```python
from build123d import *

# Parameters (mm, degrees)
SKETCH1_R                      = 127
BASE_OF_BASE_DEPTH             = 8.89
BALL_BEARING_CUT_REACH         = 221.212
SKETCH8_R                      = 26.035
SUPPORT_REACH                  = 208.429
SUPPORTS_COUNT                 = 4
CUT_FOR_PRINTABIITY_REACH      = 221.212
HOLDER_START                   = 76.2
SKETCH14_R                     = 26.035
SKETCH14_R_2                   = 13.335
HOLDER_FOR_SHOULDER_DEPTH      = 76.2
CENTER_CYLINDER_REACH          = 208.429
SKETCH14_3_R                   = 31.75
SKETCH14_3_R_2                 = 26.035
FUNNEL_INTO_SNAP_IN_PLACE_SIZE = 2.54
ACCESSIBILITY_CUT_DEPTH        = 290.1712073


with BuildPart() as part:
    # Sketch1 → Base of base (new body)
    with BuildSketch(Plane(origin=(0, 0, 0), x_dir=(1, 0, 0), z_dir=(0, 1, 0))):
        with Locations(Location((0, 0, 0), (0, 0, 270))):
            Circle(SKETCH1_R)
    extrude(amount=BASE_OF_BASE_DEPTH)



with BuildPart() as body_2:
    # Sketch7 → Top Part of Base (revolve)
    with BuildSketch(Plane(origin=(0, 0, 0), x_dir=(0, 0, -1), z_dir=(1, 0, 0)), mode=Mode.PRIVATE) as top_part_of_base_sk:
        Polygon((0, 125.681135768), (0, 112.981135768), (-114.3, 46.99), (-114.3, 59.69), align=None)
    revolve(top_part_of_base_sk.sketch.rotate(Axis((0, 8.89, 0), (0, 1, 0)), 180), axis=Axis((0, 8.89, 0), (0, 1, 0)))

    # Ball Bearing Cut: up to this cone (the profile starts outside it)
    ball_bearing_cut_end = Plane(origin=(0, 125.681136, 0), z_dir=(0, -1, 0)).offset(12.700001232) * Cone(1.732e-06, 362.01940299, 209.011998768, align=(Align.CENTER, Align.CENTER, Align.MIN), mode=Mode.PRIVATE)
    # Sketch8 → Ball Bearing Cut (cut, up to the surface)
    with BuildSketch(Plane(origin=(0, 125.681135768, 0), x_dir=(1, 0, 0), z_dir=(0, 1, 0)), mode=Mode.PRIVATE) as ball_bearing_cut_sk1:
        with Locations(Location((0, 0, 0), (0, 0, 90))):
            Circle(SKETCH8_R)
    ball_bearing_cut_tool1 = extrude(ball_bearing_cut_sk1.sketch, amount=-BALL_BEARING_CUT_REACH, mode=Mode.PRIVATE) - ball_bearing_cut_end
    add(ball_bearing_cut_tool1.solids().sort_by_distance((0, 125.681136, 0))[0], mode=Mode.SUBTRACT)


with BuildPart() as part_1:
    add(part.part)

    add(body_2.part)  # Support merges body 2
    # Support: up to this cone (the profile starts inside it)
    support_end = Plane(origin=(0, 8.89, 0), z_dir=(0, -1, 0)).offset(-104.091134768) * Cone(1.732e-06, 854.440186248, 493.311270537, align=(Align.CENTER, Align.CENTER, Align.MIN), mode=Mode.PRIVATE)
    # Sketch10 → Support (add, up to the surface)
    with BuildSketch(Plane(origin=(0, 8.89, 0), x_dir=(1, 0, 0), z_dir=(0, 1, 0)), mode=Mode.PRIVATE) as support_sk1:
        with BuildLine():
            ThreePointArc((-8.301584497, 94.887544993), (-4.154746647, 95.159343106), (0, 95.25))
            Line((0, 95.25), (0, 114.3))
            ThreePointArc((0, 114.3), (-4.985695976, 114.191211727), (-9.961901396, 113.865053992))
            Line((-9.961901396, 113.865053992), (-8.301584497, 94.887544993))
        make_face()
    support_tool1 = extrude(support_sk1.sketch, amount=SUPPORT_REACH, mode=Mode.PRIVATE) & support_end
    # Sketch10 → Support (add, up to the surface)
    with BuildSketch(Plane(origin=(0, 8.89, 0), x_dir=(1, 0, 0), z_dir=(0, 1, 0)), mode=Mode.PRIVATE) as support_sk2:
        with BuildLine():
            Line((0, 114.3), (0, 95.25))
            ThreePointArc((0, 95.25), (4.154746647, 95.159343106), (8.301584497, 94.887544993))
            Line((8.301584497, 94.887544993), (9.961901396, 113.865053992))
            ThreePointArc((9.961901396, 113.865053992), (4.985695976, 114.191211727), (0, 114.3))
        make_face()
    support_tool2 = extrude(support_sk2.sketch, amount=SUPPORT_REACH, mode=Mode.PRIVATE) & support_end
    support = support_tool1.solids().sort_by_distance((-4.581357, 8.89, -104.930336))[0] + support_tool2.solids().sort_by_distance((4.581357, 8.89, -104.930336))[0]
    add(support)

    # Supports: Support ×4 about axis
    supports_axis = Axis((0, 8.89, 0), (0, 1, 0))
    for i in range(1, SUPPORTS_COUNT):
        add(support.rotate(supports_axis, i * 360 / SUPPORTS_COUNT))

    # Cut for Printabiity: up to this cone (the profile starts outside it)
    cut_for_printabiity_end = Plane(origin=(0, 125.681136, 0), z_dir=(0, -1, 0)).offset(12.700001232) * Cone(1.732e-06, 362.01940299, 209.011998768, align=(Align.CENTER, Align.CENTER, Align.MIN), mode=Mode.PRIVATE)
    # Sketch12 → Cut for Printabiity (cut, up to the surface)
    with BuildSketch(Plane(origin=(0, 125.681135768, 0), x_dir=(1, 0, 0), z_dir=(0, 1, 0)), mode=Mode.PRIVATE) as cut_for_printabiity_sk1:
        with BuildLine():
            ThreePointArc((-113.865053992, -9.961901396), (-40.394430205, -40.394430205), (-9.961901396, -113.865053992))
            ThreePointArc((-9.961901396, -113.865053992), (-80.82230509, -80.82230509), (-113.865053992, -9.961901396))
        make_face()
    cut_for_printabiity_tool1 = extrude(cut_for_printabiity_sk1.sketch, amount=-CUT_FOR_PRINTABIITY_REACH, mode=Mode.PRIVATE) - cut_for_printabiity_end
    add(cut_for_printabiity_tool1.solids().sort_by_distance((-60.814886, 125.681136, 60.814886))[0], mode=Mode.SUBTRACT)
    # Sketch12 → Cut for Printabiity (cut, up to the surface)
    with BuildSketch(Plane(origin=(0, 125.681135768, 0), x_dir=(1, 0, 0), z_dir=(0, 1, 0)), mode=Mode.PRIVATE) as cut_for_printabiity_sk2:
        with BuildLine():
            ThreePointArc((-9.961901396, 113.865053992), (-40.394430205, 40.394430205), (-113.865053992, 9.961901396))
            ThreePointArc((-113.865053992, 9.961901396), (-80.82230509, 80.82230509), (-9.961901396, 113.865053992))
        make_face()
    cut_for_printabiity_tool2 = extrude(cut_for_printabiity_sk2.sketch, amount=-CUT_FOR_PRINTABIITY_REACH, mode=Mode.PRIVATE) - cut_for_printabiity_end
    add(cut_for_printabiity_tool2.solids().sort_by_distance((-60.814886, 125.681136, -60.814886))[0], mode=Mode.SUBTRACT)
    # Sketch12 → Cut for Printabiity (cut, up to the surface)
    with BuildSketch(Plane(origin=(0, 125.681135768, 0), x_dir=(1, 0, 0), z_dir=(0, 1, 0)), mode=Mode.PRIVATE) as cut_for_printabiity_sk3:
        with BuildLine():
            ThreePointArc((9.961901396, 113.865053992), (40.394430205, 40.394430205), (113.865053992, 9.961901396))
            ThreePointArc((113.865053992, 9.961901396), (80.82230509, 80.82230509), (9.961901396, 113.865053992))
        make_face()
    cut_for_printabiity_tool3 = extrude(cut_for_printabiity_sk3.sketch, amount=-CUT_FOR_PRINTABIITY_REACH, mode=Mode.PRIVATE) - cut_for_printabiity_end
    add(cut_for_printabiity_tool3.solids().sort_by_distance((60.814886, 125.681136, -60.814886))[0], mode=Mode.SUBTRACT)
    # Sketch12 → Cut for Printabiity (cut, up to the surface)
    with BuildSketch(Plane(origin=(0, 125.681135768, 0), x_dir=(1, 0, 0), z_dir=(0, 1, 0)), mode=Mode.PRIVATE) as cut_for_printabiity_sk4:
        with BuildLine():
            ThreePointArc((9.961901396, -113.865053992), (40.394430205, -40.394430205), (113.865053992, -9.961901396))
            ThreePointArc((113.865053992, -9.961901396), (80.82230509, -80.82230509), (9.961901396, -113.865053992))
        make_face()
    cut_for_printabiity_tool4 = extrude(cut_for_printabiity_sk4.sketch, amount=-CUT_FOR_PRINTABIITY_REACH, mode=Mode.PRIVATE) - cut_for_printabiity_end
    add(cut_for_printabiity_tool4.solids().sort_by_distance((60.814886, 125.681136, 60.814886))[0], mode=Mode.SUBTRACT)

    # Sketch14 → Holder for Shoulder (add)
    with BuildSketch(Plane(origin=(0, 8.89, 0), x_dir=(1, 0, 0), z_dir=(0, 1, 0)).offset(HOLDER_START)):
        with Locations(Location((0, 0, 0), (0, 0, 90))):
            Circle(SKETCH14_R)
        with Locations(Location((0, 0, 0), (0, 0, 90))):
            Circle(SKETCH14_R_2, mode=Mode.SUBTRACT)
    extrude(amount=-HOLDER_FOR_SHOULDER_DEPTH)

    # Center Cylinder: up to this cone (the profile starts inside it)
    center_cylinder_end = Plane(origin=(0, 8.89, 0), z_dir=(0, -1, 0)).offset(-104.091134768) * Cone(1.732e-06, 854.440186248, 493.311270537, align=(Align.CENTER, Align.CENTER, Align.MIN), mode=Mode.PRIVATE)
    # Sketch14<3> → Center Cylinder (add, up to the surface)
    with BuildSketch(Plane(origin=(0, 8.89, 0), x_dir=(1, 0, 0), z_dir=(0, 1, 0)), mode=Mode.PRIVATE) as center_cylinder_sk1:
        with Locations(Location((0, 0, 0), (0, 0, 90))):
            Circle(SKETCH14_3_R)
        with Locations(Location((0, 0, 0), (0, 0, 270))):
            Circle(SKETCH14_3_R_2, mode=Mode.SUBTRACT)
    center_cylinder_tool1 = extrude(center_cylinder_sk1.sketch, amount=CENTER_CYLINDER_REACH, mode=Mode.PRIVATE) & center_cylinder_end
    add(center_cylinder_tool1.solids().sort_by_distance((0, 8.89, 30.851974))[0])

    # Funnel into Snap in Place
    funnel_into_snap_in_place_edges = [part_1.edges().sort_by_distance(p)[0] for p in [
        (0, 85.09, 13.335),
    ]]
    chamfer(funnel_into_snap_in_place_edges, length=FUNNEL_INTO_SNAP_IN_PLACE_SIZE)

    # Sketch19 → Accessibility Cut (cut, through all)
    with BuildSketch(Plane(origin=(-61.913477694, 0, 61.913477694), x_dir=(-0.7071067811865487, 0, -0.7071067811865465), z_dir=(0.7071067811865465, 0, -0.7071067811865487))):
        Polygon((0, 8.89), (15.875, 8.89), (15.875, 43.815), (0, 59.69), (-15.875, 43.815), (-15.875, 8.89), align=None)
    extrude(amount=ACCESSIBILITY_CUT_DEPTH, mode=Mode.SUBTRACT)

    # Sketch20 → Cut-Revolve1 (revolve, cut)
    with BuildSketch(Plane(origin=(0, 0, 0), x_dir=(0, 0, -1), z_dir=(1, 0, 0))):
        Polygon((13.335, 74.295), (13.335, 79.375), (15.875, 79.375), align=None)
    revolve(axis=Axis((0, 8.89, 0), (0, 1, 0)), mode=Mode.SUBTRACT)


solid = part_1.part
```
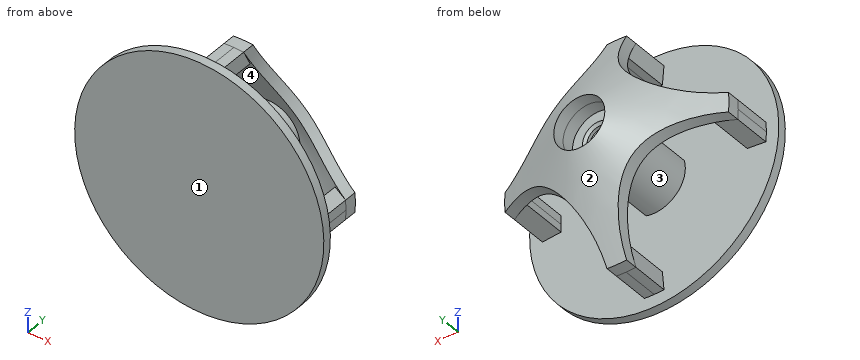
Geometry: final body of the model. Coordinates: model frame, mm. Face numbers are marked on the shaded views. Round coordinates to 2 decimals unless told otherwise and drop trailing zeros. Write each loop counter-clockwise with the first axis right and the second up, starting at its lowest first coordinate (ties: lowest second). Pieces come first, ordered by that corner, then holes.
Item 1: Section query A-A (y = 36). Return loops of the section in (x, z), plus the area to 3 significant figures.
Item 2: Pin query (flat end, axial travel): P1, Ø1, axis at x = -75.5, z = 57, coming from the +Y side; P2, Ø10, axis at x = -27.5, z = -76.5, coming from the -Y side; P3, Ø3, axis at y = 60.5, z = 1, coming from the -X side; P4, Ø1.5, axis at y = 36, z = -93, coming from the -X side. Return the tip coordinate at first contact, or that it passes through.
Item 3: Mould query, pull axis Z, two halves, no side actions, for the marked faces 1, 2, 3 and 4. Classes: +Z half, -Z half, draft (parallel to the pull), parting line (faces both ways), or undercut.
Item 4: Material intervals for L1, parallel to Y at x = -63, z = -84; L2, parallel to X at y = 81, z = 0 (3 decimals); L3, parallel to X at y = 67.25, z = 0 (3 decimals), sorted ascending.
Completed:
1. outline: (-113.87, -9.96) - (-94.89, -8.3) arc R95.25 cw to (-94.89, 8.3) - (-113.87, 9.96) arc R114.3 ccw to start; (-30.67, 8.22) arc R31.75 ccw to (8.22, -30.67) - close; (-9.96, -113.87) arc R114.3 ccw to (9.96, -113.87) - (8.3, -94.89) arc R95.25 cw to (-8.3, -94.89) - close; (-9.96, 113.87) - (-8.3, 94.89) arc R95.25 cw to (8.3, 94.89) - (9.96, 113.87) arc R114.3 ccw to start; (-8.22, 30.67) - (30.67, -8.22) arc R31.75 ccw to start; (94.89, -8.3) - (113.87, -9.96) arc R114.3 ccw to (113.87, 9.96) - (94.89, 8.3) arc R95.25 cw to start
1. area: 2,630 mm2
2. P1: stops at y = 8.89
2. P2: stops at y = 0
2. P3: stops at x = -114.3
2. P4: passes through
3. face 1: draft
3. face 2: parting line
3. face 3: undercut
3. face 4: undercut
4. L1: y = 0 to 8.89
4. L2: x = -77.39 to -55.393, -31.75 to -13.335, 13.335 to 31.75, 55.393 to 77.39
4. L3: x = -101.206 to -79.209, -31.75 to -13.335, 13.335 to 31.75, 79.209 to 101.206
